Could you check a few things on this model? Use its own coordinates, in mm. A direction names the side the tool comes from. Give positions to 0.01 mm unless a question says otherwise; leave off trailing zeros. Order: outer loops, then holes, each group sorted by start corner. A loop starts at its lowest first (then second) coordinate and runs counter-clockwise, first axis right, second up. Notation, with made-up numbers: M 85,-21.75 L 137,-21.75 A17 cw 137,11.25 Z; hole C -16,9 d4. An arc over 180 degrees is marked long. Use a Markdown table: item, result. Add a question column.
Item 1: Suppose I cut it at B-B on y = -0.65. Count the separate pieces of the cut face and the enclosed holes in it, plus the area to 3 significant figures.
Item 2: I'm going to push flat-ended pins straight in: pin 1 Ø6.5 at (x, z) = (-12.5, 12.5) entering from -Y; pin 2 Ø0.6 at (y, z) = (-0.5, 26.5) entering from -X. Where does each tip first touch, or does it pass through?
Item 3: If I drill on L1, parallel to Z at x = -25.5, y = -1.45; L2, parallel to X at y = -1.5, z = 26; L3, parallel to Z at x = 7.5, y = -1.8, over which ranges is the centre line in solid material (lowest first)? Write a range as from..to.
Item 4: For faces 5 (the face through (12.5, -1, 26)), 6 (the face through (0, -1, 37.5)), which set-ups out of +Z, -Z, +X, -X, +Y, -Y let a thin tool reach every point of the face, with its end or its side?
Item 5: If we mould it in two halves opening along Z, with no side actions, what happens to faces 1 (the face through (12, -1, 29)), 2 (the face through (0, -1, 22)), 3 (the face through (33.89, -1.01, 34.08)), 4 (the face through (-1, -2, -1))? For each: released by +Z, released by -Z, zero draft, split by the parting line, or undercut.
Item 6: Suppose I cut it at A-A on z = 11.5. Write out the boundary of the cut face in (x, y).
from build123d import *

# Parameters (mm, degrees)
SKETCH_1_W             = 75
SKETCH_1_H             = 75
SKETCH_1_R             = 6
SKETCH_1_R_2           = 2
SKETCH_1_W_2           = 8
SKETCH_1_H_2           = 25
SKETCH_1_W_3           = 25
SKETCH_1_H_3           = 8
SM_BASE_FLANGE_1_DEPTH = 2
FILLET_1_R             = 12
FILLET_2_R             = 2.5


# Sheet-metal steps are written as plain solids
with BuildPart() as part:
    # Sketch 1 → 基体-法兰1 (new body)
    with BuildSketch(Plane(origin=(0, 0, 0), x_dir=(1, 0, 0), z_dir=(0, 1, 0))):
        Rectangle(SKETCH_1_W, SKETCH_1_H)
        with Locations(Location((26, 26, 0), (0, 0, 270))):
            Circle(SKETCH_1_R, mode=Mode.SUBTRACT)
        with Locations(Location((26, -26, 0), (0, 0, 270))):
            Circle(SKETCH_1_R, mode=Mode.SUBTRACT)
        with Locations(Location((-26, -26, 0), (0, 0, 270))):
            Circle(SKETCH_1_R, mode=Mode.SUBTRACT)
        with Locations(Location((-26, 26, 0), (0, 0, 270))):
            Circle(SKETCH_1_R, mode=Mode.SUBTRACT)
        with Locations(Location((-12.5, 12.5, 0), (0, 0, 270))):
            Circle(SKETCH_1_R_2, mode=Mode.SUBTRACT)
        with Locations(Location((12.5, 12.5, 0), (0, 0, 270))):
            Circle(SKETCH_1_R_2, mode=Mode.SUBTRACT)
        with Locations(Location((12.5, -12.5, 0), (0, 0, 270))):
            Circle(SKETCH_1_R_2, mode=Mode.SUBTRACT)
        with Locations(Location((-12.5, -12.5, 0), (0, 0, 270))):
            Circle(SKETCH_1_R_2, mode=Mode.SUBTRACT)
        with Locations((26, 0)):
            Rectangle(SKETCH_1_W_2, SKETCH_1_H_2, mode=Mode.SUBTRACT)
        with Locations((0, 26)):
            Rectangle(SKETCH_1_W_3, SKETCH_1_H_3, mode=Mode.SUBTRACT)
        with Locations((0, -26)):
            Rectangle(SKETCH_1_W_3, SKETCH_1_H_3, mode=Mode.SUBTRACT)
        with Locations((-26, 0)):
            Rectangle(SKETCH_1_W_2, SKETCH_1_H_2, mode=Mode.SUBTRACT)
    extrude(amount=-SM_BASE_FLANGE_1_DEPTH)

    # 圆角1
    fillet_1_edges = [part.edges().sort_by_distance(p)[0] for p in [
        (-37.5, -1, -37.5),
        (37.5, -1, -37.5),
        (37.5, -1, 37.5),
        (-37.5, -1, 37.5),
    ]]
    fillet(fillet_1_edges, radius=FILLET_1_R)

    # 圆角2
    fillet_2_edges = [part.edges().sort_by_distance(p)[0] for p in [
        (-12.5, -1, -22),
        (-12.5, -1, -30),
        (12.5, -1, -30),
        (12.5, -1, -22),
        (30, -1, -12.5),
        (30, -1, 12.5),
        (22, -1, 12.5),
        (22, -1, -12.5),
        (12.5, -1, 30),
        (-12.5, -1, 30),
        (-12.5, -1, 22),
        (12.5, -1, 22),
        (-30, -1, 12.5),
        (-30, -1, -12.5),
        (-22, -1, -12.5),
        (-22, -1, 12.5),
    ]]
    fillet(fillet_2_edges, radius=FILLET_2_R)


solid = part.part
Findings below:
| question | item | result |
|---|---|---|
| 1 | separate pieces | 1 |
| 1 | enclosed holes | 12 |
| 1 | area | 4,220 mm^2 |
| 2 | pin 1 | stops at y = -2 |
| 2 | pin 2 | stops at x = -37.48 |
| 3 | L1 | z = -37.5..-31.98, -20.02..-12.5, 12.5..20.02, 31.98..37.5 |
| 3 | L2 | x = -37.49..-32, -20..-12.5, 12.5..20, 32..37.49 |
| 3 | L3 | z = -37.5..-30, -22..22, 30..37.5 |
| 4 | face 5 | +Y, -Y |
| 4 | face 6 | +Z, +X, -X, +Y, -Y |
| 5 | face 1 | undercut |
| 5 | face 2 | undercut |
| 5 | face 3 | released by +Z |
| 5 | face 4 | zero draft |
| 6 | outline | M -37.5,-2 L -29.5,-2 L -29.5,0 L -37.5,0 Z; M -22.5,-2 L -14.23,-2 L -14.23,0 L -22.5,0 Z; M -10.77,-2 L 10.77,-2 L 10.77,0 L -10.77,0 Z; M 14.23,-2 L 22.5,-2 L 22.5,0 L 14.23,0 Z; M 29.5,-2 L 37.5,-2 L 37.5,0 L 29.5,0 Z |
